from build123d import *

# Parameters (mm, degrees)
SKETCH034_R      = 1
SKETCH034_W      = 12.5
SKETCH034_H      = 2.25
EXTRUDE032_DEPTH = 2
SKETCH033_W      = 47.5
SKETCH033_H      = 36
EXTRUDE031_DEPTH = 2


with BuildPart() as extrude032:
    # Sketch034 → Extrude032 (new body)
    with BuildSketch(Plane.XY.offset(-0.5)):
        with Locations((155.15, 11.2)):
            Circle(SKETCH034_R)
        with Locations((155.15, 26.45)):
            Circle(SKETCH034_R)
        with Locations((151.25, 30.225)):
            Rectangle(SKETCH034_W, SKETCH034_H)
    extrude(amount=-EXTRUDE032_DEPTH)


with BuildPart() as sensorsheet:
    # Sketch033 → Extrude031 (new body)
    with BuildSketch(Plane.XY.offset(1.5)):
        with Locations((151.25, 26.5)):
            Rectangle(SKETCH033_W, SKETCH033_H)
    extrude(amount=-EXTRUDE031_DEPTH)

    # Fusion009: union Extrude032
    add(extrude032.part)


solid = sensorsheet.part
Build history of the part. All positions in model axes, mm. A direction names the side the tool comes from. Round coordinates to 2 decimals unless told otherwise and drop trailing zeros. Write each loop counter-clockwise with the first axis right and the second up, starting at its lowest first coordinate (ties: lowest second). Pieces come first, ordered by that corner, then holes. Notation, with made-up numbers: (-25, 71.5) -> (29, 71.5) arc R34 cw to (29, 107.5) -> close; hole circle Ø3 at (75, -16.75). An arc over 180 degrees is marked (long way). Write item = value, one per line.
(1) Band-saw the part on C-C (x = 163). Give the cut face in (y, z), then the cut area to 3 significant figures.
Answer:
outline = (8.5, -0.5) -> (44.5, -0.5) -> (44.5, 1.5) -> (8.5, 1.5) -> close
area = 72.0 mm2
(2) Band-saw the part on A-A (x = 153). Give the cut face in (y, z), then the cut area to 3 significant figures.
Answer:
outline = (8.5, -0.5) -> (29.1, -0.5) -> (29.1, -2.5) -> (31.35, -2.5) -> (31.35, -0.5) -> (44.5, -0.5) -> (44.5, 1.5) -> (8.5, 1.5) -> close
area = 76.5 mm2
(3) Flat gauge pins, fed straight in: pin 1 (1 mm diameter, centred on x = 150, z = -2, fed in from +Y); pin 2 (4 mm diameter, centred on x = 169, y = 18, fed in from -Z); pin 3 (1.6 mm diameter, centred on x = 149.5, z = -2, fed in from -Y). Where does each tip first touch, or does it go through?
Answer:
pin_1 = 31.35
pin_2 = -0.5
pin_3 = 29.1
(4) Probe L1, parallel to Z at x = 137, y = 21; L2, parallel to X at y = 26.5, z = -1.2; L3, parallel to X at y = 30, z = -0.55. List the from-to ranges inside material, lowest first.
Answer:
L1 = -0.5 to 1.5
L2 = 154.15 to 156.15
L3 = 145 to 157.5
(5) Band-saw the part on D-D (y = 36). Give the cut face in (x, z).
Answer:
outline = (127.5, -0.5) -> (175, -0.5) -> (175, 1.5) -> (127.5, 1.5) -> close
(6) Band-saw the part on B-B (y = 26.45). Give the cut face in (x, z).
Answer:
outline = (127.5, -0.5) -> (154.15, -0.5) -> (154.15, -2.5) -> (156.15, -2.5) -> (156.15, -0.5) -> (175, -0.5) -> (175, 1.5) -> (127.5, 1.5) -> close
(7) Tool access for faces 1 (the face through (145, 30, -1)), 2 (the face through (151, 8.5, 1)), 3 (the face through (157.5, 30, -1)): list every direction of +Z, -Z, +X, -X, +Y, -Y with a clear straight run to the whole face (end or side of a thin tool).
Answer:
face_1 = -Z, -X, +Y, -Y
face_2 = +Z, -Z, +X, -X, -Y
face_3 = -Z, +X, +Y, -Y
(8) Two-plate mould, pull along Y, no slides. Class faces 4 (the face through (154.15, 11.24, -1.49)), 5 (the face through (154.36, 25.84, -1.49)), 6 (the face through (151, 27, 1.5)), 7 (the face through (151, 31.35, -1)): pulls with the +Y half, pulls with the -Y half, needs draft (parallel to the pull), parting line crosses it, or undercut.
Answer:
face_4 = undercut
face_5 = undercut
face_6 = needs draft
face_7 = pulls with the +Y half
